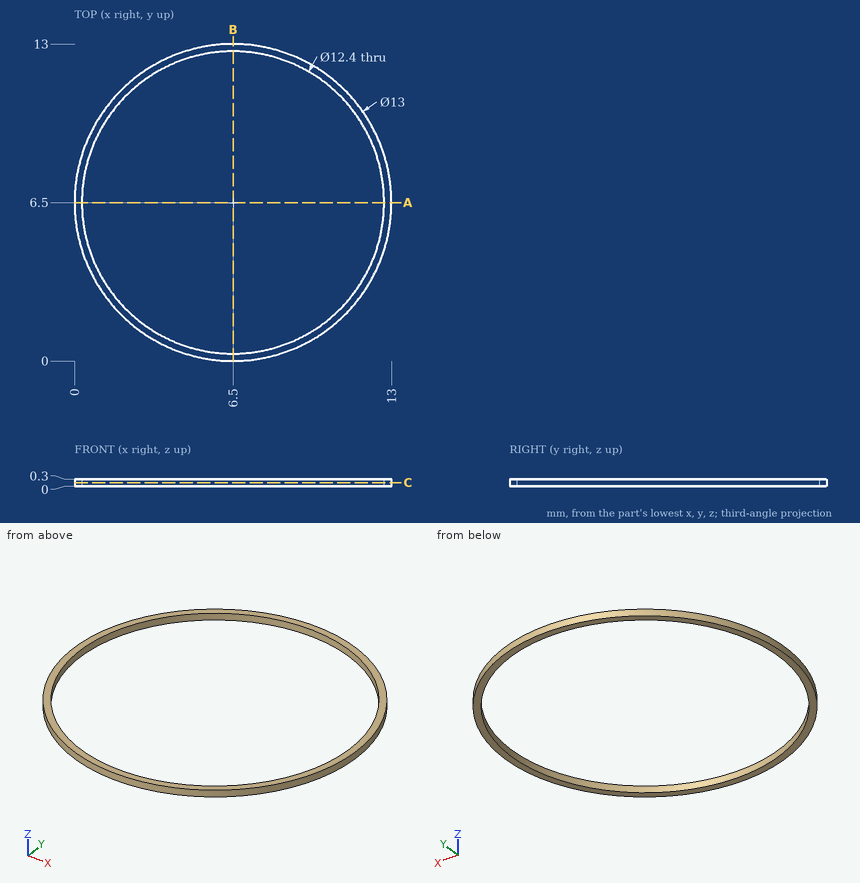
Design review of the part shown in the three views and the two pictorial views. Dimensions are in mm from the part's minimum x, y and z. Round coordinates to 2 decimals unless told otherwise and drop trailing zeros. Order: outer loops, then holes, each group sorted by start corner. A loop starts at its lowest first (then second) coordinate and runs counter-clockwise, first axis right, second up. Notation, with made-up numbers: (30.5, 22.5) -> (75.5, 22.5) arc R8 cw to (75.5, 29.5) -> close; hole circle Ø5 at (88.25, -6). An arc over 180 degrees is marked (long way). Write item = value, one per line. Start each with the question number.
1) Take a section at C-C on z = 0.15. State the section outline as (x, y) points.
2) To check wall thickness, follow line 1 (Y direction, x = 6.5, z = 0.1); line 2 (Y direction, x = 3, z = 0.2); line 3 (X direction, y = 10.5, z = 0.2). State the ranges of each line that lie inside material, in increasing order. Write a range as from..to.
3) Take a section at A-A on y = 6.5. State the section outline as (x, z) points, plus the area to 3 significant figures.
Verdict:
q1.outline = circle Ø13 at (6.5, 6.5); hole circle Ø12.4 at (6.5, 6.5)
q2.line_1 = 0..0.3, 12.7..13
q2.line_2 = 1.02..1.38, 11.62..11.98
q2.line_3 = 1.38..1.76, 11.24..11.62
q3.outline = (0, 0) -> (0.3, 0) -> (0.3, 0.3) -> (0, 0.3) -> close; (12.7, 0) -> (13, 0) -> (13, 0.3) -> (12.7, 0.3) -> close
q3.area = 0.180 mm2
